CAD build for the part. Positions are in the model's coordinates, mm. A direction names the side the tool comes from. Give positions to 0.01 mm unless a question says otherwise; leave off trailing zeros. Loops run counter-clockwise (first coordinate to the right, second up) from the corner with the lowest first, then second, coordinate; pieces in that order, holes last. Notation, with made-up numbers: (20.5, 9.5) - (56.5, 9.5) arc R29 cw to (56.5, 31.5) - close; hole circle Ø5 at (82.5, 65.25). An arc over 180 degrees is marked (long way). Return JSON: item names as keys, results as strings.
from build123d import *

# Parameters (mm, degrees)
SKETCH1_R           = 6.35
BOSS_EXTRUDE1_DEPTH = 73.533


with BuildPart() as part:
    # Sketch1 → Boss-Extrude1 (new, symmetric)
    with BuildSketch(Plane(origin=(0, 0, 0), x_dir=(1, 0, 0), z_dir=(0, 1, 0))):
        with Locations(Location((0, 0, 0), (0, 0, 270))):
            Circle(SKETCH1_R)
    extrude(amount=BOSS_EXTRUDE1_DEPTH, both=True)

    # Sketch2 → #10-32 Tapped Hole1 (revolve, cut)
    with BuildSketch(Plane(origin=(0, 73.533, 0), x_dir=(0, 0, 1), z_dir=(1, 0, 0))):
        Polygon((0, 0), (0, 13.151317848), (2.0193, 11.938), (2.0193, 0), align=None)
    f_10_32_tapped_hole1 = revolve(axis=Axis((0, 79.883, 0), (0, -1, 0)), mode=Mode.SUBTRACT)

    # Mirror1: #10-32 Tapped Hole1 across plane
    add(f_10_32_tapped_hole1.mirror(Plane.ZX), mode=Mode.SUBTRACT)


solid = part.part
1. Cut at C-C, the plane x = -5. Write the cut outline in (y, z), plus the area to 3 significant figures.
Values follow:
{"outline": "(-73.53, -3.91) - (73.53, -3.91) - (73.53, 3.91) - (-73.53, 3.91) - close", "area": "1,150 mm²"}
2. Cut at A-A, the plane y = 63. Write the cut outline in (x, z), plus the area to 3 significant figures.
Values follow:
{"outline": "circle Ø12.7 at (0, 0); hole circle Ø4.04 at (0, 0)", "area": "114 mm²"}
3. Drill centre lines: probe 1 along X at (y, z) = (66.5, 0); probe 2 along Z at (x, y) = (-4.5, 55.5); probe 3 along X at (y, z) = (56.5, -3.75). Where is each one in solid material? Low to high.
Values follow:
{"probe 1": "x = -6.35 to -2.02, 2.02 to 6.35", "probe 2": "z = -4.48 to 4.48", "probe 3": "x = -5.12 to 5.12"}
4. Cut at B-B, the plane z = 3.75. Write the cut outline in (x, y), plus the area to 3 significant figures.
Values follow:
{"outline": "(-5.12, -73.53) - (5.12, -73.53) - (5.12, 73.53) - (-5.12, 73.53) - close", "area": "1,510 mm²"}
5. Pull direction X, two halves, no side cores. Call faces 3 (the face through (2, -73.533, -2)), 4 (the face through (-3.86, 1.03, -5.04)), 5 (the face through (-0.607, -67.648, 1.926)): +X half, -X half, draft (parallel to the pull), parting line (faces both ways), or undercut.
Values follow:
{"face 3": "draft", "face 4": "parting line", "face 5": "undercut"}
6. Drop flat-ended pins along their axis: P1, Ø5, axis at y = 44, z = 5, coming from the -X side; P2, Ø1, axis at x = 1.5, y = -24.5, coming from the +Z side; P3, Ø6.5, axis at x = 0, z = 0, coming from the -Y side; P4, Ø3, axis at x = 0, z = 0, coming from the -Y side. Give the stop position or say it passes through.
Values follow:
{"P1": "stops at x = -5.84", "P2": "stops at z = 6.27", "P3": "stops at y = -73.53", "P4": "stops at y = -61.28"}
7. Which spindle directions (+Z, -Z, +X, -X, +Y, -Y) get a long thin tool onto all of the face, cutting with end or side? Do faces 1 (the face through (-0.607, 67.648, 1.926)), 2 (the face through (2, 73.533, -2)). Say none if no direction does.
Values follow:
{"face 1": "+Y", "face 2": "+Z, -Z, +X, -X, +Y"}
